Check sheet for the modelled part. Datum: model origin and axes. Units: mm. A direction names the side the tool comes from. Coordinates: 2 decimals unless noted, no trailing zeros. Write each loop counter-clockwise with the first axis right and the second up, starting at its lowest first coordinate (ties: lowest second). Pieces come first, ordered by that corner, then holes. Notation, with made-up numbers: M 20,-13 L 45,-13 A8 cw 45,-2 Z; hole C -39,-8.75 d3. An arc over 180 degrees is marked long. Answer as CSV lines item,"result".
Autodesk Inventor part; units mm, degrees
ref_plane "YZ Plane" through (0, 0, 0) normal (1, 0, 0) x (0, 1, 0)
ref_plane "XZ Plane" through (0, 0, 0) normal (0, 1, 0) x (-1, 0, 0)
ref_plane "XY Plane" through (0, 0, 0) normal (0, 0, 1) x (1, 0, 0)
sketch "Sketch1" plane through (0, 0, 0) normal (0, 1, 0) x (-1, 0, 0)
  line L0 (10, -12) -> (-10, -12)
  line L1 (-12, -10) -> (-12, 10)
  line L2 (-10, 12) -> (10, 12)
  line L3 (12, 10) -> (12, -10)
  line L4 (12, -12) -> (-12, 12) construction
  line L5 (-12, -12) -> (12, 12) construction
  line L6 (8.4853, -8.4853) -> (6.7353, -8.4853)
  line L7 (-8.4853, -8.4853) -> (-8.4853, -6.7353)
  line L8 (-8.4853, 8.4853) -> (-6.7353, 8.4853)
  line L9 (8.4853, 8.4853) -> (8.4853, 6.7353)
  line L10 (8.4853, -8.4853) -> (-8.4853, 8.4853) construction
  line L11 (-8.4853, -8.4853) -> (8.4853, 8.4853) construction
  circle A0 centre (-8.4853, 8.4853) radius 1.75
  circle A1 centre (8.4853, 8.4853) radius 1.75
  circle A2 centre (-8.4853, -8.4853) radius 1.75
  circle A3 centre (8.4853, -8.4853) radius 1.75
  line L12 (-10, 12) -> (-12, 10)
  line L13 (-12, -10) -> (-10, -12)
  line L14 (10, -12) -> (12, -10)
  line L15 (10, 12) -> (12, 10)
  line L16 (-6.7353, 8.4853) -> (6.7353, 8.4853)
  line L17 (6.7353, 8.4853) -> (8.4853, 8.4853)
  line L18 (-8.4853, 6.7353) -> (-8.4853, 8.4853)
  line L19 (-8.4853, -6.7353) -> (-8.4853, 6.7353)
  line L20 (-6.7353, -8.4853) -> (-8.4853, -8.4853)
  line L21 (6.7353, -8.4853) -> (-6.7353, -8.4853)
  line L22 (8.4853, -6.7353) -> (8.4853, -8.4853)
  line L23 (8.4853, 6.7353) -> (8.4853, -6.7353)
  point P0 (0, 0)
  dimension "d0" = 24
  dimension "d1" = 24
  dimension "d2" = 12
  dimension "d3" = 3.5
  dimension "d4" = 3.5
  dimension "d5" = 3.5
  dimension "d6" = 3.5
  dimension "d7" = 2
  dimension "d8" = 2
  dimension "d9" = 2
  dimension "d10" = 2
  dimension "d11" = 2
  dimension "d12" = 2
  dimension "d13" = 2
  dimension "d14" = 2
extrude "Extrusion1" add sketch "Sketch1" along normal blind 5 contours L0 L13 L1 L12 L2 L15 L3 L14 | L21 A2 L19 A0 L16 A1 L23 A3
sketch "Sketch2" plane through (0, 5, 0) normal (0, 1, 0) x (1, 0, 0)
  circle A0 centre (0, 0) radius 6
  dimension "d17" = 12
extrude "Extrusion2" add sketch "Sketch2" along normal blind 40
sketch "Sketch3" plane through (0, 45, 0) normal (0, 1, 0) x (1, 0, 0)
  circle A0 centre (0, 0) radius 6
  circle A1 centre (0, 0) radius 4
  dimension "d20" = 8
extrude "Extrusion3" cut sketch "Sketch3" against normal through all contours A1
equation "\"d8\" = d7"
equation "\"d9\" = d7"
equation "\"d10\" = d9"
equation "\"d11\" = d7"
equation "\"d12\" = d11"
equation "\"d13\" = d7"
equation "\"d14\" = d13"
properties part number "lm8kuu"
1) Mould release check, pull along X, two halves, no side actions. Record for faces 3 (the face through (8.71, 2.46, -10.22)), 4 (the face through (11, 2, 11)), 5 (the face through (3, 0, 3)): pulls with the +X half, pulls with the -X half, needs draft (parallel to the pull), parting line crosses it, or undercut.
Answer key:
face 3,"undercut"
face 4,"pulls with the +X half"
face 5,"needs draft"
2) Section check B-B, the plane z = 9.25. Record the boundary of the cut face in (x, y).
Answer key:
outline,"M -12,0 L -10.06,0 L -10.06,5 L -12,5 Z; M -6.91,0 L 6.91,0 L 6.91,5 L -6.91,5 Z; M 10.06,0 L 12,0 L 12,5 L 10.06,5 Z"
3) Tool access check on faces 1 (the face through (-6, 25, 0)), 2 (the face through (12, 2, 0)). Record the directions out of +Z, -Z, +X, -X, +Y, -Y that give a thin tool (end or side, any length) a straight path to the whole face; none if there is none.
Answer key:
face 1,"+Y"
face 2,"+Z, -Z, +X, +Y, -Y"
4) Section check A-A, the plane x = 0. Record the boundary of the cut face in (y, z), plus the area to 3 significant figures.
Answer key:
outline,"M 0,-12 L 5,-12 L 5,-6 L 45,-6 L 45,-4 L 0,-4 Z; M 0,4 L 45,4 L 45,6 L 5,6 L 5,12 L 0,12 Z"
area,"240 mm2"
5) Thickness scan on line 1 along Z through (x, y) = (-0.25, 40); line 2 along X through (y, z) = (31.5, -2.5); line 3 along Y through (x, z) = (-3.25, -9). Record the ranges inside material, lowest first.
Answer key:
line 1,"z = -5.99 to -3.99, 3.99 to 5.99"
line 2,"x = -5.45 to -3.12, 3.12 to 5.45"
line 3,"y = 0 to 5"
6) Depth check by flat-ended pin: P1, Ø12, axis at x = -6.5, y = 12.5, coming from the -Z side; P2, Ø3, axis at x = 8.49, z = -8.49, coming from the +Y side; P3, Ø6, axis at x = 5, y = 9, coming from the -Z side; P4, Ø3, axis at y = 11, z = -4, coming from the +X side. Enter the tip coordinate at first touch or a pass-through.
Answer key:
P1,"stops at z = -5.98"
P2,"passes through"
P3,"stops at z = -5.66"
P4,"stops at x = 5.45"
7) Section check D-D, the plane x = -8.5. Record the boundary of the cut face in (y, z).
Answer key:
outline,"M 0,-12 L 5,-12 L 5,-10.24 L 0,-10.24 Z; M 0,-6.74 L 5,-6.74 L 5,6.74 L 0,6.74 Z; M 0,10.24 L 5,10.24 L 5,12 L 0,12 Z"
8) Section check C-C, the plane z = 0. Record the boundary of the cut face in (x, y).
Answer key:
outline,"M -12,0 L -4,0 L -4,45 L -6,45 L -6,5 L -12,5 Z; M 4,0 L 12,0 L 12,5 L 6,5 L 6,45 L 4,45 Z"
